Design review of the part built by this model. Coordinates are the model's own, in mm. Face numbers are marked on the shaded views. A direction names the side the tool comes from. Give positions to 0.01 mm unless a question says otherwise; leave off trailing zeros. Order: outer loops, then holes, each group sorted by start corner. A loop starts at its lowest first (then second) coordinate and runs counter-clockwise, first axis right, second up. Notation, with made-up numbers: M 59.25,46.25 L 75.25,46.25 A25 cw 75.25,72.25 Z; hole C 19,43.25 d6. An arc over 180 degrees is marked long. Answer as a JSON object with one key per item and string values.
from build123d import *

# Parameters (mm, degrees)
SKETCH_1_W           = 46
SKETCH_1_H           = 20
EXTRUDE_1_DEPTH      = 12
SKETCH_2_R           = 8.25
CUT_EXTRUDE_1_DEPTH  = 13
SKETCH_3_W           = 8
SKETCH_3_H           = 6
CUT_EXTRUDE_2_DEPTH  = 13
SKETCH_4_W           = 5
SKETCH_4_H           = 4
CUT_EXTRUDE_3_DEPTH  = 13
SKETCH_5_W           = 3
SKETCH_5_H           = 2
SKETCH_5_W_2         = 2
SKETCH_5_H_2         = 3
CUT_EXTRUDE_4_DEPTH  = 1
SKETCH_6_W           = 46
SKETCH_6_H           = 12
EXTRUDE_2_DEPTH      = 15
SKETCH_14_R          = 1.6
CUT_EXTRUDE_10_DEPTH = 46
SKETCH_15_R          = 2.25
CUT_EXTRUDE_11_DEPTH = 13
SKETCH1_R            = 1.6
CUT_EXTRUDE1_DEPTH   = 13
SKETCH2_R            = 4
CUT_EXTRUDE2_DEPTH   = 2
CHAMFER1_SIZE        = 0.5
CHAMFER2_SIZE        = 0.5


with BuildPart() as part:
    # 草圖1 → 填料-伸長1 (new body)
    with BuildSketch(Plane.XY):
        Rectangle(SKETCH_1_W, SKETCH_1_H)
    extrude(amount=EXTRUDE_1_DEPTH)

    # 草圖2 → 除料-伸長1 (cut, through all)
    with BuildSketch(Plane.XY.offset(12)):
        with Locations((-12.7, -0.65)):
            Circle(SKETCH_2_R)
        with Locations((12.7, -0.65)):
            Circle(SKETCH_2_R)
    extrude(amount=-CUT_EXTRUDE_1_DEPTH, mode=Mode.SUBTRACT)

    # 草圖3 → 除料-伸長2 (cut, through all)
    with BuildSketch(Plane.XY.offset(12)):
        with Locations((0, 7)):
            Rectangle(SKETCH_3_W, SKETCH_3_H)
    extrude(amount=-CUT_EXTRUDE_2_DEPTH, mode=Mode.SUBTRACT)

    # 草圖4 → 除料-伸長3 (cut, through all)
    with BuildSketch(Plane.XY.offset(12)):
        with Locations((0, -5.5)):
            Rectangle(SKETCH_4_W, SKETCH_4_H)
    extrude(amount=-CUT_EXTRUDE_3_DEPTH, mode=Mode.SUBTRACT)

    # 草圖5 → 除料-伸長4 (cut)
    with BuildSketch(Plane.XY.offset(12)):
        with Locations((4, -6.5)):
            Rectangle(SKETCH_5_W, SKETCH_5_H)
        with Locations((-5.5, 8)):
            Rectangle(SKETCH_5_W_2, SKETCH_5_H_2)
        with Locations((5.5, 8)):
            Rectangle(SKETCH_5_W_2, SKETCH_5_H_2)
    extrude(amount=-CUT_EXTRUDE_4_DEPTH, mode=Mode.SUBTRACT)

    # 草圖6 → 填料-伸長2 (add)
    with BuildSketch(Plane.XZ.offset(10)):
        with Locations((0, 6)):
            Rectangle(SKETCH_6_W, SKETCH_6_H)
    extrude(amount=EXTRUDE_2_DEPTH)

    # 草圖14 → 除料-伸長10 (cut)
    with BuildSketch(Plane.XY.offset(12)):
        with Locations((-21, 8)):
            Circle(SKETCH_14_R)
    extrude(amount=-CUT_EXTRUDE_10_DEPTH, mode=Mode.SUBTRACT)

    # 草圖15 → 除料-伸長11 (cut, through all)
    with BuildSketch(Plane(origin=(0, 0, 0), x_dir=(-1, 0, 0), z_dir=(0, 0, -1))):
        with Locations((-15, -18)):
            Circle(SKETCH_15_R)
        with Locations((15, -18)):
            Circle(SKETCH_15_R)
    extrude(amount=-CUT_EXTRUDE_11_DEPTH, mode=Mode.SUBTRACT)

    # Sketch1 → Cut-Extrude1 (cut, through all)
    with BuildSketch(Plane.XY.offset(12)):
        with Locations((20, -10)):
            Circle(SKETCH1_R)
    extrude(amount=-CUT_EXTRUDE1_DEPTH, mode=Mode.SUBTRACT)

    # Sketch2 → Cut-Extrude2 (cut)
    with BuildSketch(Plane.XY.offset(12)):
        with Locations((-15, -18)):
            Circle(SKETCH2_R)
        with Locations((15, -18)):
            Circle(SKETCH2_R)
    extrude(amount=-CUT_EXTRUDE2_DEPTH, mode=Mode.SUBTRACT)

    # Chamfer1
    chamfer1_edges = [part.edges().sort_by_distance(p)[0] for p in [
        (-23, 10, 6),
        (23, 10, 6),
    ]]
    chamfer(chamfer1_edges, length=CHAMFER1_SIZE)

    # Chamfer2
    chamfer2_edges = [part.edges().sort_by_distance(p)[0] for p in [
        (-23, -25, 6),
        (23, -25, 6),
    ]]
    chamfer(chamfer2_edges, length=CHAMFER2_SIZE)


solid = part.part
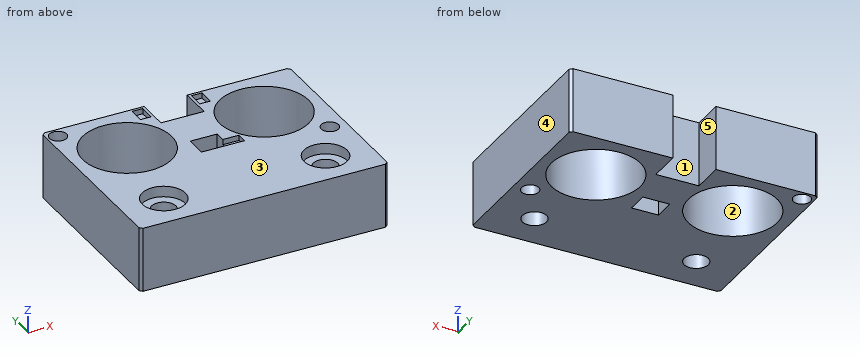
(1) Insertion check: pin 1 (1.5 mm diameter, centred on x = -17, y = -16, fed in from +Z); pin 2 (1.9 mm diameter, centred on x = -21, y = 8, fed in from +Z). Each pin has a flat end and moves straight along its axis. Give the tip position at first contact, or say it passes through.
Checked values:
{"pin 1": "stops at z = 10", "pin 2": "passes through"}
(2) Tool access review of the marked faces 4 and 5: name each direction out of +Z, -Z, +X, -X, +Y, -Y from which nothing blocks a thin tool from reaching the whole face with its end or side.
Checked values:
{"face 4": "+Z, -Z, +X, +Y, -Y", "face 5": "+Z, -Z, +Y"}
(3) Draft analysis for pull direction Y (two halves, no side actions). For the marked faces 1, 2 and 3, state which applies: +Y half, -Y half, draft (parallel to the pull), parting line (faces both ways), or undercut.
Checked values:
{"face 1": "+Y half", "face 2": "undercut", "face 3": "draft"}
(4) We need section D-D (z = 9.5). Write out the cut boundary in (x, y), plus the area to 3 significant figures.
Checked values:
{"outline": "M -23,-24.5 L -22.5,-25 L 22.5,-25 L 23,-24.5 L 23,9.5 L 22.5,10 L 4,10 L 4,4 L -4,4 L -4,10 L -22.5,10 L -23,9.5 Z; hole C -21,8 d3.2; hole C -12.7,-0.65 d16.5; hole C -15,-18 d4.5; hole M -2.5,-7.5 L 2.5,-7.5 L 2.5,-3.5 L -2.5,-3.5 Z; hole C 12.7,-0.65 d16.5; hole C 15,-18 d4.5; hole C 20,-10 d3.2", "area": "1,070 mm^2"}
(5) We need section C-C (y = -10). Write out the cut boundary in (x, z), plus the area to 3 significant figures.
Checked values:
{"outline": "M -23,0 L 18.4,0 L 18.4,12 L -23,12 Z; M 21.6,0 L 23,0 L 23,12 L 21.6,12 Z", "area": "514 mm^2"}
(6) To check wall thickness, follow L1, parallel to Y at x = 12.7, z = 7; L2, parallel to Y at x = 20, z = 6.5; L3, parallel to X at y = 2.5, z = 10.5. State the ranges of each line that lie inside material, in increasing order. Write a range as from..to.
Checked values:
{"L1": "y = -25..-8.9, 7.6..10", "L2": "y = -25..-11.6, -8.4..-4.49, 3.19..10", "L3": "x = -23..-20.32, -5.08..5.08, 20.32..23"}
(7) We need section B-B (y = -0.65). Write out the cut boundary in (x, z), plus the area to 3 significant figures.
Checked values:
{"outline": "M -23,0 L -20.95,0 L -20.95,12 L -23,12 Z; M -4.45,0 L 4.45,0 L 4.45,12 L -4.45,12 Z; M 20.95,0 L 23,0 L 23,12 L 20.95,12 Z", "area": "156 mm^2"}
(8) We need section A-A (x = 0). Write out the cut boundary in (y, z), plus the area to 3 significant figures.
Checked values:
{"outline": "M -25,0 L -7.5,0 L -7.5,12 L -25,12 Z; M -3.5,0 L 4,0 L 4,12 L -3.5,12 Z", "area": "300 mm^2"}
